Check sheet for the drawn part. Datum: minimum x, y, z corner. Units: mm. A direction names the side the tool comes from. Give positions to 0.01 mm unless a question says otherwise; leave off trailing zeros. Loops run counter-clockwise (first coordinate to the right, second up) from the corner with the lowest first, then second, coordinate; pieces in that order, holes last. Notation, with made-up numbers: (37.5, -26.5) - (47.5, -26.5) arc R31 cw to (47.5, 2.5) - close; hole circle Ø7 at (21.5, 43). An arc over 180 degrees is marked (long way). Use one line per item in the form item = value.
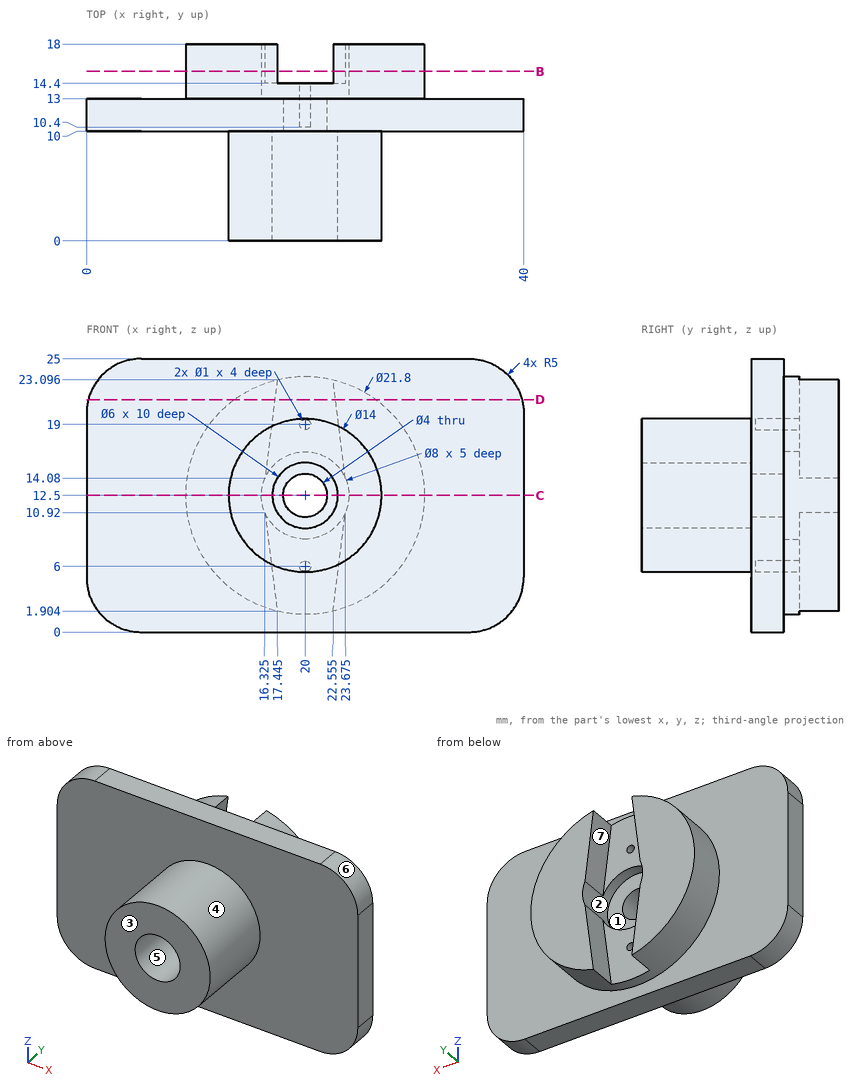
Item 1: Section check B-B on y = 15.5. Record the boundary of the cut face in (x, z) (1 decimal).
Answer block:
outline = (16.3, 10.9) arc R4 cw to (16.3, 14.1) - (17.4, 23.1) arc R10.9 ccw to (17.4, 1.9) - close; (22.6, 1.9) arc R10.9 ccw to (22.6, 23.1) - (23.7, 14.1) arc R4 cw to (23.7, 10.9) - close
Item 2: Access from +Z, -Z, +X, -X, +Y, -Y to the whole of each face (thin tool, end or side, straight path). Record for the marked faces 5, 6 and 7.
Answer block:
face_5 = -Y
face_6 = +Z, +X, +Y, -Y
face_7 = +Y
Item 3: Section check D-D on z = 21.25. Record the boundary of the cut face in (x, y) (1 decimal), then the cut area to 3 significant figures.
Answer block:
outline = (0.2, 10) - (39.8, 10) - (39.8, 13) - (26.5, 13) - (26.5, 18) - (22.8, 18) - (22.8, 14.4) - (17.2, 14.4) - (17.2, 18) - (13.5, 18) - (13.5, 13) - (0.2, 13) - close
area = 164 mm2
Item 4: Mould release check, pull along X, two halves, no side actions. Record for the marked faces 1, 2, 3 and 4: released by +X, released by -X, zero draft, split by the parting line, or undercut.
Answer block:
face_1 = undercut
face_2 = undercut
face_3 = zero draft
face_4 = split by the parting line
Item 5: Section check C-C on z = 12.5. Record the boundary of the cut face in (x, y), then the cut area to 3 significant figures.
Answer block:
outline = (0, 10) - (13, 10) - (13, 0) - (17, 0) - (17, 10) - (18, 10) - (18, 13) - (16, 13) - (16, 18) - (9.1, 18) - (9.1, 13) - (0, 13) - close; (22, 10) - (23, 10) - (23, 0) - (27, 0) - (27, 10) - (40, 10) - (40, 13) - (30.9, 13) - (30.9, 18) - (24, 18) - (24, 13) - (22, 13) - close
area = 257 mm2
Item 6: Thickness scan on L1, parallel to X at y = 12.5, z = 6; L2, parallel to X at y = 6.5, z = 12.5; L3, parallel to Y at x = 28, z = 15.75. Record the ranges inside material, lowest first.
Answer block:
L1 = 0 to 19.5, 20.5 to 40
L2 = 13 to 17, 23 to 27
L3 = 10 to 18
Item 7: Gauge pin test, flat ends, axial feed: P1, Ø1.8, axis at x = 21.5, z = 13.5, coming from the -Y side; P2, Ø4.5, axis at x = 20, z = 12.5, coming from the +Y side; P3, Ø6, axis at x = 19, y = 6, coming from the +Z side. Record the tip position at first contact, or that the pin passes through.
Answer block:
P1 = 10
P2 = 13
P3 = 19.5
